from build123d import *

# Parameters (mm, degrees)
F2_SIZE  = 2
F3_SIZE  = 2
F4_W     = 8
F4_H     = 6.6
F5_DEPTH = 37.401
F6_R     = 3.4
F7_DEPTH = 62.501
F8_R     = 3.4
F9_DEPTH = 62.501
F10_SIZE = 1
F11_SIZE = 2


with BuildPart() as f1:
    # F0 (on Right) → F1 (revolve)
    with BuildSketch(Plane.YZ):
        with BuildLine():
            Line((-12.7, 62.5), (-12.7, 12.5))
            Line((-12.7, 12.5), (12.7, 12.5))
            Line((12.7, 12.5), (24.7, 12.5))
            Line((24.7, 12.5), (24.7, 30))
            Line((24.7, 30), (12.7, 30))
            Line((12.7, 30), (12.7, 62.5))
            Line((12.7, 62.5), (7.969316, 62.5))
            ThreePointArc((7.969316, 62.5), (7.332673, 62.271159), (6.98741, 61.689373))
            Line((6.98741, 61.689373), (3.96875, 46.0375))
            Line((3.96875, 46.0375), (0, 46.0375))
            Line((0, 46.0375), (-3.96875, 46.0375))
            Line((-3.96875, 46.0375), (-6.98741, 61.689373))
            ThreePointArc((-6.98741, 61.689373), (-7.332673, 62.271159), (-7.969316, 62.5))
            Line((-7.969316, 62.5), (-12.7, 62.5))
        make_face()
    revolve(axis=Axis((0, -1.982494, 0), (0, 1, 0)))

    # F2
    f2_edges = [f1.edges().sort_by_distance(p)[0] for p in [
        (0, 12.7, -62.5),
    ]]
    chamfer(f2_edges, length=F2_SIZE)

    # F3
    f3_edges = [f1.edges().sort_by_distance(p)[0] for p in [
        (0, -12.7, -62.5),
    ]]
    chamfer(f3_edges, length=F3_SIZE)

    # F4 (on face) → F5 (cut, through all)
    with BuildSketch(Plane(origin=(0, 24.7, 0), x_dir=(-1, 0, 0), z_dir=(0, 1, 0))):
        with Locations((0, 12.5)):
            Rectangle(F4_W, F4_H)
    extrude(amount=-F5_DEPTH, mode=Mode.SUBTRACT)

    # F6 (on Top) → F7 (cut, through all)
    with BuildSketch(Plane.XY):
        with Locations((0, 18.7)):
            Circle(F6_R)
    extrude(amount=F7_DEPTH, mode=Mode.SUBTRACT)

    # F8 (on Right) → F9 (cut, through all)
    with BuildSketch(Plane.YZ):
        with Locations((18.7, 0)):
            Circle(F8_R)
    extrude(amount=-F9_DEPTH, mode=Mode.SUBTRACT)

    # F10
    f10_edges = [f1.edges().sort_by_distance(p)[0] for p in [
        (0, 24.7, -12.5),
        (0, -12.7, -12.5),
    ]]
    chamfer(f10_edges, length=F10_SIZE)

    # F11
    f11_edges = [f1.edges().sort_by_distance(p)[0] for p in [
        (0, 24.7, -30),
    ]]
    chamfer(f11_edges, length=F11_SIZE)


solid = f1.part
Could you check a few things on this model? Use its own coordinates, in mm. A direction names the side the tool comes from. Give positions to 0.01 mm unless a question says otherwise; leave off trailing zeros. Order: outer loops, then holes, each group sorted by start corner. A loop starts at its lowest first (then second) coordinate and runs counter-clockwise, first axis right, second up. Notation, with made-up numbers: (-29.75, 49) - (-11.75, 49) arc R28 cw to (-11.75, 80) - close; hole circle Ø1 at (-18, -39.5). An arc over 180 degrees is marked (long way). One line per item, written item: value. Start each with the question number.
1. For P1, Ø12, axis at y = 19.5, z = -5, coming from the -X side; P2, Ø6, axis at y = 0.5, z = 40.5, coming from the +X side; P3, Ø4.5, axis at y = 8, z = 13.5, coming from the -X side, each with a flat end and sliding along its axis, tell me the tip position at first contact or that it passes through.
2. If I drill on probe 1 along Y at (x, z) = (0, 20); probe 2 along X at (y, z) = (-3, -0.5); probe 3 along X at (y, z) = (14, 0), over which ranges is the centre line in solid material (lowest first)?
3. Imagine slicing it at A-A on y = 2.5. List the corners of the cut face in (x, z) for me (1 decimal).
4. Imagine slicing it at B-B on z = 0. Give the number of separate pieces and of enclosed holes in the cut face, plus the area to 3 significant figures.
5. Imagine slicing it at D-D on y = 18.7. List the corners of the cut face in (x, z) for me, plus the area to 3 significant figures.
6. For faces 4 (the face through (-0.74, 15.38, 22.8)), 5 (the face through (-28.013, -0.056, -36.534)), 6 (the face through (4, 6, 14)), 7 (the face through (-20.883, 21.943, 1.021)), 8 (the face through (1.32, 17.63, -29.97)), which set-ups out of +Z, -Z, +X, -X, +Y, -Y let a thin tool reach every point of the face, with its end or its side?
7. Thinking about a two-plate mould opening in X: for faces 1 (the face through (-28.476, 4.115, -37.137)), 2 (the face through (-12, 24.7, 7)), 3 (the face through (0.5, 23.87, -12.66)), which applies, +X half, -X half, draft (parallel to the pull), parting line (faces both ways), or undercut?
Values:
1. P1: x = -30
1. P2: x = 26.71
1. P3: x = -61.48
2. probe 1: -12.7 to 15.3, 22.1 to 24.7
2. probe 2: -46.03 to -12.49, 12.49 to 46.03
2. probe 3: -30 to -12.5, 12.5 to 30
3. outline: circle Ø92.1 at (0, 0); hole (-4, 11.8) arc R12.5 ccw (long way) to (4, 11.8) - (4, 15.8) - (-4, 15.8) - close
4. separate pieces: 3
4. enclosed holes: 0
4. area: 2,460 mm²
5. outline: (-29.81, -3.4) arc R30 ccw (long way) to (3.4, 29.81) - (3.4, 15.8) - (4, 15.8) - (4, 11.84) arc R12.5 cw (long way) to (-12.03, -3.4) - close; (-29.81, 3.4) - (-12.03, 3.4) arc R12.5 cw to (-4, 11.84) - (-4, 15.8) - (-3.4, 15.8) - (-3.4, 29.81) arc R30 ccw to start
5. area: 2,090 mm²
6. face 4: +Z
6. face 5: none
6. face 6: +Y, -Y
6. face 7: -X
6. face 8: +Y
7. face 1: parting line
7. face 2: draft
7. face 3: undercut
